Work out the finished part from the listing and answer in its coordinate system (mm). Face numbers are marked on the shaded views. A direction names the side the tool comes from. Round coordinates to 2 decimals unless told otherwise and drop trailing zeros. Order: outer loops, then holes, each group sorted by start corner. A loop starts at its lowest first (then second) coordinate and runs counter-clockwise, first axis right, second up. Notation, with made-up numbers: (21, 16) - (29, 16) arc R25 cw to (29, 37) - close; hole circle Ø7 at (26.5, -9). An arc over 180 degrees is marked (long way). Answer in a Markdown table with one row per item.
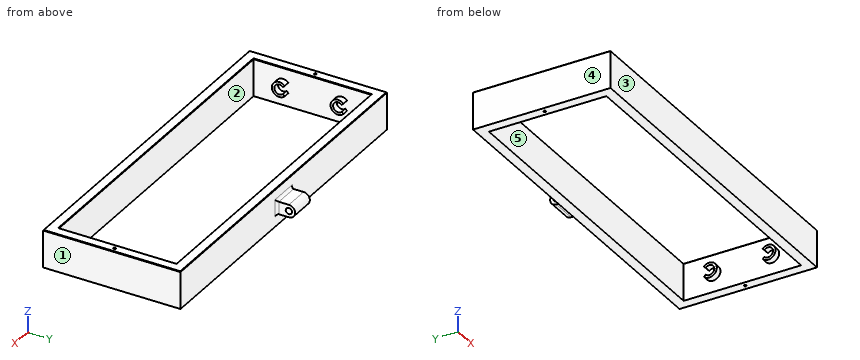
from build123d import *

# Parameters (mm, degrees)
SKETCH1_W                                = 140
SKETCH1_H                                = 55
SKETCH1_W_2                              = 132
SKETCH1_H_2                              = 47
RECTANGLE_PAD_DEPTH                      = 15
MOUNTINGHOLES_DEPTH                      = 2.5
TAP_DRILL_FOR_M1_2X0_25_TAP2_D           = 0.95
TAP_DRILL_FOR_M1_2X0_25_TAP2_CSINK_D     = 1
TAP_DRILL_FOR_M1_2X0_25_TAP2_CSINK_ANGLE = 90
CHAMFER3_SIZE                            = 0.2
BOSS_EXTRUDE1_DEPTH                      = 10
FILLET1_R                                = 1
SKETCH7_R                                = 1.25
CUT_EXTRUDE1_DEPTH                       = 10


with BuildPart() as part:
    # Sketch1 → Rectangle Pad (new body)
    with BuildSketch(Plane.XY):
        Rectangle(SKETCH1_W, SKETCH1_H)
        Rectangle(SKETCH1_W_2, SKETCH1_H_2, mode=Mode.SUBTRACT)
    extrude(amount=RECTANGLE_PAD_DEPTH)

    # Sketch2 → MountingHoles (add)
    with BuildSketch(Plane.ZY.offset(-66)):
        with BuildLine():
            Line((8.875, 13.202368755), (9.582283213, 13.909651968))
            ThreePointArc((9.582283213, 13.909651968), (7.5, 8.75), (5.417716787, 13.909651968))
            Line((5.417716787, 13.909651968), (6.125, 13.202368755))
            ThreePointArc((6.125, 13.202368755), (7.5, 9.75), (8.875, 13.202368755))
        make_face()
        with BuildLine():
            Line((8.875, -10.297631245), (9.582283213, -9.590348032))
            ThreePointArc((9.582283213, -9.590348032), (7.5, -14.75), (5.417716787, -9.590348032))
            Line((5.417716787, -9.590348032), (6.125, -10.297631245))
            ThreePointArc((6.125, -10.297631245), (7.5, -13.75), (8.875, -10.297631245))
        make_face()
    mountingholes = extrude(amount=MOUNTINGHOLES_DEPTH)

    # Mirror1: MountingHoles across plane
    add(mountingholes.mirror(Plane(origin=(0, 0, 0), x_dir=(0, 0, 1), z_dir=(1, 0, 0))))

    # Tap Drill for M1.2x0.25 Tap2 (through all)
    with Locations(Plane.XY.offset(15)):
        with Locations((68, 0), (-68, 0)):
            CounterSinkHole(TAP_DRILL_FOR_M1_2X0_25_TAP2_D / 2, TAP_DRILL_FOR_M1_2X0_25_TAP2_CSINK_D / 2, counter_sink_angle=TAP_DRILL_FOR_M1_2X0_25_TAP2_CSINK_ANGLE)

    # Chamfer3
    chamfer3_edges = [part.edges().sort_by_distance(p)[0] for p in [
        (-70, 0, 15),
        (66, 0, 15),
        (0, -27.5, 15),
        (0, 23.5, 15),
        (-66, 0, 15),
        (0, -23.5, 15),
        (70, 0, 15),
        (0, 27.5, 15),
    ]]
    chamfer(chamfer3_edges, length=CHAMFER3_SIZE)

    # Sketch6 → Boss-Extrude1 (add)
    with BuildSketch(Plane(origin=(-5, 0, 0), x_dir=(0, 0, -1), z_dir=(1, 0, 0))):
        with BuildLine():
            Line((-9.9, 32.5), (-9.9, 27.5))
            Line((-9.9, 27.5), (-4.9, 27.5))
            Line((-4.9, 27.5), (-4.9, 32.5))
            ThreePointArc((-4.9, 32.5), (-7.4, 35), (-9.9, 32.5))
        make_face()
    extrude(amount=BOSS_EXTRUDE1_DEPTH)

    # Fillet1
    fillet1_edges = [part.edges().sort_by_distance(p)[0] for p in [
        (-5, 27.5, 7.4),
        (0, 27.5, 9.9),
        (0, 27.5, 4.9),
        (5, 27.5, 7.4),
    ]]
    fillet(fillet1_edges, radius=FILLET1_R)

    # Sketch7 → Cut-Extrude1 (cut)
    with BuildSketch(Plane.ZY.offset(5)):
        with Locations((7.4, 32.5)):
            Circle(SKETCH7_R)
    extrude(amount=-CUT_EXTRUDE1_DEPTH, mode=Mode.SUBTRACT)


solid = part.part
1) The mould has two halves that part along Y. Classify the marked faces 1, 2 and 3: released by +Y, released by -Y, zero draft, split by the parting line, or undercut.
Filled in:
| item | result |
|---|---|
| face 1 | zero draft |
| face 2 | undercut |
| face 3 | released by -Y |
2) Find section B-B, the plane y = 11.75. Give the vertices of the cut face in (x, z), then the cut area to 3 significant figures.
Filled in:
| item | result |
|---|---|
| outline | (-70, 0) - (-66, 0) - (-66, 4.5) - (-63.5, 4.5) - (-63.5, 5.5) - (-66, 5.5) - (-66, 9.5) - (-63.5, 9.5) - (-63.5, 10.5) - (-66, 10.5) - (-66, 14.8) - (-66.2, 15) - (-69.8, 15) - (-70, 14.8) - close; (63.5, 4.5) - (66, 4.5) - (66, 0) - (70, 0) - (70, 14.8) - (69.8, 15) - (66.2, 15) - (66, 14.8) - (66, 10.5) - (63.5, 10.5) - (63.5, 9.5) - (66, 9.5) - (66, 5.5) - (63.5, 5.5) - close |
| area | 130 mm^2 |
3) Find section C-C, the plane x = -14. Give the vertices of the cut face in (y, z), then the cut area to 3 significant figures.
Filled in:
| item | result |
|---|---|
| outline | (-27.5, 0) - (-23.5, 0) - (-23.5, 14.8) - (-23.7, 15) - (-27.3, 15) - (-27.5, 14.8) - close; (23.5, 0) - (27.5, 0) - (27.5, 14.8) - (27.3, 15) - (23.7, 15) - (23.5, 14.8) - close |
| area | 120 mm^2 |
4) Which of the six approach directions +Z, -Z, +X, -X, +Y, -Y give full straight-line access (tool end or side, diameter ignored) to the marked faces 4 and 5?
Filled in:
| item | result |
|---|---|
| face 4 | +Z, -Z, -X, +Y, -Y |
| face 5 | +Z, -Z |
5) Each of these flat-tipped pins is pushed along its axis until it touches: pin 1 (2 mm diameter, centred on x = 35, z = 3.5, fed in from +Y); pin 2 (2 mm diameter, centred on x = 0.5, y = 30, fed in from +Z); pin 3 (1.5 mm diameter, centred on y = 33, z = 6.5, fed in from -X). Where does it stop, or does it pass through?
Filled in:
| item | result |
|---|---|
| pin 1 | stops at y = 27.5 |
| pin 2 | stops at z = 9.9 |
| pin 3 | stops at x = -5 |
6) Find section A-A, the plane x = 3.5. Give the vertices of the cut face in (y, z).
Filled in:
| item | result |
|---|---|
| outline | (-27.5, 0) - (-23.5, 0) - (-23.5, 14.8) - (-23.7, 15) - (-27.3, 15) - (-27.5, 14.8) - close; (23.5, 0) - (27.5, 0) - (27.5, 3.9) arc R1 cw to (28.5, 4.9) - (32.5, 4.9) arc R2.5 ccw to (32.5, 9.9) - (28.5, 9.9) arc R1 cw to (27.5, 10.9) - (27.5, 14.8) - (27.3, 15) - (23.7, 15) - (23.5, 14.8) - close; hole circle Ø2.5 at (32.5, 7.4) |
7) Find section D-D, the plane z = 12.25. Give the vertices of the cut face in (x, y) (3 decimals), then the cut area to 3 significant figures.
Filled in:
| item | result |
|---|---|
| outline | (-70, -27.5) - (70, -27.5) - (70, 27.5) - (-70, 27.5) - close; hole circle Ø0.95 at (-68, 0); hole (-66, -23.5) - (66, -23.5) - (66, 23.5) - (-66, 23.5) - close; hole circle Ø0.95 at (68, 0) |
| area | 1,490 mm^2 |
8) Find the intervals of material crossed by probe 1 along Y at (x, z) = (1, 7.4); probe 2 along Y at (x, z) = (64.05, 7.5); probe 3 along X at (y, z) = (20, 3.5), in increasing order. Write a range as from..to.
Filled in:
| item | result |
|---|---|
| probe 1 | y = -27.5..-23.5, 23.5..31.25, 33.75..35 |
| probe 2 | y = -27.5..-23.5, -14.75..-13.75, 8.75..9.75, 23.5..27.5 |
| probe 3 | x = -70..-66, 66..70 |
